Can you work these out from the model? Positions are in its coordinate system, mm. A direction names the side the tool comes from. Round coordinates to 2 decimals unless told otherwise and drop trailing zeros. Order: outer loops, then holes, each group sorted by start corner. A loop starts at its lowest first (then second) coordinate and runs counter-clockwise, first axis right, second up.
Q1. We'd pull the mould along Y, two halves only. Please class faces 1 (the face through (30.88, -15.32, -15.62)), 2 (the face through (9.2, 18, 18)), 3 (the face through (34.964, -16.881, -21.094)): pulls with the +Y half, pulls with the -Y half, needs draft (parallel to the pull), parting line crosses it, or undercut.
Q2. If we section it at C-C (y = 0): Please give me the cut outline in (x, z).
Q3. For faces 4 (the face through (19.898, 21.102, 14.032)), 5 (the face through (9.2, 18, -18)), 6 (the face through (19.898, -21.102, -14.032)), 7 (the face through (40.49, 9.98, -5.19)), which set-ups out of +Z, -Z, +X, -X, +Y, -Y let a thin tool reach every point of the face, with its end or its side?
Q4. If we section it at D-D (x = 56.5): Please give me the cut outline in (y, z).
Q5. If I drill on line 1 (Y direction, x = 37.5, z = -15.5); line 2 (Z direction, x = 4, y = -15), over which ranges is the centre line in solid material (lowest first)?
Q6. If we section it at B-B (z = 0): Please give me the cut outline in (x, y).
Q7. If we section it at A-A (x = 37): Please give me the cut outline in (y, z).
Q8. Will these pins go through, and if not, where does the flat tip stop? P1, Ø4, axis at y = -15.5, z = -15.5, coming from the +X side; P2, Ø2.5, axis at y = 17, z = -17.5, coming from the -X side; P3, Ø1.5, axis at y = -15.5, z = 15.5, coming from the +X side; P4, Ø3.5, axis at x = 3, z = -26, coming from the -Y side.
Autodesk Inventor part; units mm, degrees
ref_plane "YZ Plane" through (0, 0, 0) normal (1, 0, 0) x (0, 1, 0)
ref_plane "XZ Plane" through (0, 0, 0) normal (0, 1, 0) x (-1, 0, 0)
ref_plane "XY Plane" through (0, 0, 0) normal (0, 0, 1) x (1, 0, 0)
sketch "スケッチ1" plane through (0, 0, 0) normal (1, 0, 0) x (0, 1, 0)
  line L0 (-21.25, 21.25) -> (21.25, 21.25)
  line L1 (21.25, 21.25) -> (21.25, -21.25)
  line L2 (21.25, -21.25) -> (-21.25, -21.25)
  line L3 (-21.25, -21.25) -> (-21.25, 21.25)
  line L4 (-21.25, 21.25) -> (21.25, -21.25) construction
  line L5 (21.25, 21.25) -> (-21.25, -21.25) construction
  line L6 (16.9338, 21.25) -> (21.25, 16.9338)
  line L7 (21.25, -16.9338) -> (16.9338, -21.25)
  line L8 (-16.9338, -21.25) -> (-21.25, -16.9338)
  line L9 (-21.25, 16.9338) -> (-15.808, 22.3758)
  point P0 (0, 0)
  point P1 (0, 0)
  point P2 (0, 0)
  point P3 (-16.9338, 21.25)
  dimension "d0" = 42.5
  dimension "d1" = 42.5
  dimension "d2" = 27
  dimension "d3" = 27
  dimension "d4" = 27
  dimension "d5" = 27
extrude "押し出し1" add sketch "スケッチ1" along normal blind 9.2 contours L6 L1 L7 L2 L8 L3 L9 L0
sketch "スケッチ2" plane through (9.2, 0, 0) normal (1, 0, 0) x (0, 0, -1)
  line L0 (16.9338, 21.25) -> (-16.9338, 21.25)
  line L1 (-21.25, 16.9338) -> (-21.25, -16.9338)
  line L2 (-16.9338, -21.25) -> (16.9338, -21.25)
  line L3 (21.25, -16.9338) -> (21.25, 16.9338)
  line L4 (-21.25, 14.1053) -> (-14.1053, 21.25)
  line L5 (14.1053, 21.25) -> (21.25, 14.1053)
  line L6 (21.25, -14.1053) -> (14.1053, -21.25)
  line L7 (-14.1053, -21.25) -> (-21.25, -14.1053)
  point P0 (0, 0)
  dimension "d8" = 25
  dimension "d9" = 25
  dimension "d10" = 25
  dimension "d11" = 25
  dimension "d12" = 135
extrude "押し出し2" add sketch "スケッチ2" along normal blind 21.1
sketch "スケッチ3" plane through (30.3, 0, 0) normal (1, 0, 0) x (0, 0, -1)
  line L0 (-16.9338, -21.25) -> (16.9338, -21.25)
  line L1 (-21.25, -16.9338) -> (-16.9338, -21.25)
  line L2 (-21.25, 16.9338) -> (-21.25, -16.9338)
  line L3 (-16.9338, 21.25) -> (-21.25, 16.9338)
  line L4 (16.9338, 21.25) -> (-16.9338, 21.25)
  line L5 (21.25, 16.9338) -> (16.9338, 21.25)
  line L6 (21.25, -16.9338) -> (21.25, 16.9338)
  line L7 (16.9338, -21.25) -> (21.25, -16.9338)
  point P0 (0, 0)
extrude "押し出し3" add sketch "スケッチ3" along normal blind 9.2
sketch "スケッチ4" plane through (0, 0, 0) normal (-1, 0, 0) x (0, 0, 1)
  line L0 (15.5, 15.5) -> (-15.5, 15.5) construction
  line L1 (-15.5, 15.5) -> (-15.5, -15.5) construction
  line L2 (-15.5, -15.5) -> (15.5, -15.5) construction
  line L3 (15.5, -15.5) -> (15.5, 15.5) construction
  line L4 (15.5, 15.5) -> (-15.5, -15.5) construction
  line L5 (-15.5, 15.5) -> (15.5, -15.5) construction
  point P0 (0, 0)
  dimension "d17" = 31
  dimension "d18" = 31
hole "穴1" at (0, 15.5, -15.5) at (0, -15.5, -15.5) at (0, -15.5, 15.5) at (0, 15.5, 15.5) direction (1, 0, 0) diameter 2.5 depth 8 tip angle 118
chamfer "面取り1" distance 0.5 angle 45 4 edges at (0, -15.5, -16.75) (0, 15.5, -16.75) (0, -15.5, 14.25) (0, 15.5, 14.25)
thread "ねじ1"
thread "ねじ3"
thread "ねじ4"
thread "ねじ5"
sketch "スケッチ5" plane through (39.5, 0, 0) normal (1, 0, 0) x (0, 0, -1)
  line L0 (-15.5, -15.5) -> (15.5, -15.5) construction
  line L1 (15.5, -15.5) -> (15.5, 15.5) construction
  line L2 (15.5, 15.5) -> (-15.5, 15.5) construction
  line L3 (-15.5, 15.5) -> (-15.5, -15.5) construction
  line L4 (-15.5, -15.5) -> (15.5, 15.5) construction
  line L5 (15.5, -15.5) -> (-15.5, 15.5) construction
  point P0 (0, 0)
  dimension "d31" = 31
  dimension "d32" = 31
hole "穴2" at (39.5, -15.5, 15.5) at (39.5, -15.5, -15.5) at (39.5, 15.5, -15.5) at (39.5, 15.5, 15.5) direction (-1, 0, 0) diameter 2.5 depth 8 tip angle 118
chamfer "面取り2" distance 0.5 angle 45 4 edges at (39.5, -15.5, 16.75) (39.5, -15.5, -14.25) (39.5, 15.5, 16.75) (39.5, 15.5, -14.25)
thread "ねじ2"
thread "ねじ6"
thread "ねじ7"
thread "ねじ8"
sketch "スケッチ6" plane through (39.5, 0, 0) normal (1, 0, 0) x (0, 0, -1)
  circle A0 centre (0, 0) radius 11.25
  dimension "d57" = 22.5
extrude "押し出し4" add sketch "スケッチ6" along normal blind 2
sketch "スケッチ7" plane through (41.5, 0, 0) normal (1, 0, 0) x (0, 0, -1)
  circle A0 centre (0, 0) radius 2.5
  dimension "d60" = 5
extrude "押し出し5" add sketch "スケッチ7" along normal blind 19
sketch "スケッチ8" plane through (0, 0, 0) normal (-1, 0, 0) x (0, 0, 1)
  circle A0 centre (0, 0) radius 4.5
  dimension "d63" = 9
extrude "押し出し6" cut sketch "スケッチ8" against normal blind 3
sketch "スケッチ14" plane through (0, -16.9338, -21.25) normal (0, 0, -1) x (-1, 0, 0)
  line L0 (0, 0) -> (0, 33.8675)
  line L1 (-9.2, 0) -> (-9.2, 2.8284)
  line L2 (0, 8.9338) -> (-9.2, 8.9338)
  line L3 (-9.2, 8.9338) -> (-9.2, 24.9338)
  line L4 (-9.2, 24.9338) -> (0, 24.9338)
  line L5 (0, 24.9338) -> (0, 8.9338)
  point P0 (0, 16.9338)
  point P1 (-9.2, 16.9338)
  point P2 (0, 16.9338)
  point P3 (0, 16.9338)
  point P4 (0, 16.9338)
  point P5 (0, 24.9338)
  dimension "d97" = 16
extrude "押し出し10" add sketch "スケッチ14" along normal blind 7
fillet "フィレット1" radius 2 24 edges at (34.9, -16.9338, -21.25) (34.9, -21.25, -16.9338) (19.75, -14.1053, -21.25) (19.75, -21.25, -14.1053) (4.6, -16.9338, -21.25) (4.6, -21.25, -16.9338) (19.75, 14.1053, -21.25) (19.75, 21.25, -14.1053) (4.6, 21.25, -16.9338) (4.6, 16.9338, -21.25) (34.9, 16.9338, -21.25) (34.9, 21.25, -16.9338) (4.6, 21.25, 16.9338) (4.6, 16.9338, 21.25) (19.75, 14.1053, 21.25) (19.75, 21.25, 14.1053) (34.9, 21.25, 16.9338) (34.9, 16.9338, 21.25) (19.75, -14.1053, 21.25) (4.6, -16.9338, 21.25) (4.6, -21.25, 16.9338) (19.75, -21.25, 14.1053) (34.9, -16.9338, 21.25) (34.9, -21.25, 16.9338)
properties part number "stepper_motor"
Solution:
1. face 1: undercut
1. face 2: needs draft
1. face 3: pulls with the -Y half
2. outline: (0, -28.25) - (9.2, -28.25) - (9.2, -21.25) - (39.5, -21.25) - (39.5, -11.25) - (41.5, -11.25) - (41.5, -2.5) - (60.5, -2.5) - (60.5, 2.5) - (41.5, 2.5) - (41.5, 11.25) - (39.5, 11.25) - (39.5, 21.25) - (0, 21.25) - (0, 4.5) - (3, 4.5) - (3, -4.5) - (0, -4.5) - close
3. face 4: +Z, +Y
3. face 5: -Z, +Y
3. face 6: -Z, -Y
3. face 7: +X
4. outline: circle Ø5 at (0, 0)
5. line 1: y = -21.25 to -16.75, -14.25 to 14.25, 16.75 to 21.25
5. line 2: z = -21.25 to -16.65, -14.35 to 14.35, 16.65 to 21.25
6. outline: (0, -21.25) - (39.5, -21.25) - (39.5, -11.25) - (41.5, -11.25) - (41.5, -2.5) - (60.5, -2.5) - (60.5, 2.5) - (41.5, 2.5) - (41.5, 11.25) - (39.5, 11.25) - (39.5, 21.25) - (0, 21.25) - (0, 4.5) - (3, 4.5) - (3, -4.5) - (0, -4.5) - close
7. outline: (-21.25, -16.11) arc R2 ccw to (-20.66, -17.52) - (-17.52, -20.66) arc R2 ccw to (-16.11, -21.25) - (16.11, -21.25) arc R2 ccw to (17.52, -20.66) - (20.66, -17.52) arc R2 ccw to (21.25, -16.11) - (21.25, 16.11) arc R2 ccw to (20.66, 17.52) - (17.52, 20.66) arc R2 ccw to (16.11, 21.25) - (-16.11, 21.25) arc R2 ccw to (-17.52, 20.66) - (-20.66, 17.52) arc R2 ccw to (-21.25, 16.11) - close; hole circle Ø2.5 at (-15.5, -15.5); hole circle Ø2.5 at (-15.5, 15.5); hole circle Ø2.5 at (15.5, -15.5); hole circle Ø2.5 at (15.5, 15.5)
8. P1: stops at x = 39.5
8. P2: stops at x = 0
8. P3: stops at x = 31.2
8. P4: stops at y = -8
